Here's how the part is built. I have some questions about the finished solid (model axes, mm). Face numbers are marked on the shaded views. A direction names the side the tool comes from. Round coordinates to 2 decimals unless told otherwise and drop trailing zeros. Write each loop counter-clockwise with the first axis right and the second up, starting at its lowest first coordinate (ties: lowest second). Pieces come first, ordered by that corner, then holes. Notation, with made-up numbers: M -5,-27.75 L 23,-27.75 A15 cw 23,-2.75 Z; hole C -6,31 d1. An arc over 180 degrees is marked long. Use one line per item in the form item = value. Start each with the question number.
Q1. I want a section at A-A on x = -24.5. List the corners of the cut face in (y, z) for me.
Q2. I want a section at C-C on x = 5.5. List the corners of the cut face in (y, z) for me.
Q3. For the marked faces 1 and 2, which set-ups out of +Z, -Z, +X, -X, +Y, -Y let a thin tool reach every point of the face, with its end or its side?
Q4. I'm going to push flat-ended pins straight in: pin 1 Ø10 at (y, z) = (-18, 8) entering from -X; pin 2 Ø1 at (x, z) = (-18.5, 8.5) entering from +Y; pin 3 Ø10 at (x, y) = (-4.5, -1.5) entering from +Z. Where does each tip first touch, or does it pass through?
Q5. I want a section at D-D on z = 19.25. List the corners of the cut face in (x, y) for me, and give its area (3 significant figures).
Q6. I want a section at B-B on y = 1.5. List the corners of the cut face in (x, z) for me, and give its area (3 significant figures).
Q7. I need wall thicknesses on line 1 along Z through (x, y) = (-19, 15); line 2 along Y through (x, z) = (-9.5, 4). Which ranges of each line are inside material? Lowest first, please. Write a range as from..to.
```python
from build123d import *

# Parameters (mm, degrees)
SKETCH_1_W      = 40
SKETCH_1_H      = 70
EXTRUDE_1_DEPTH = 2
SKETCH_2_W      = 40
SKETCH_2_H      = 2
EXTRUDE_2_DEPTH = 20


with BuildPart() as part:
    # 草图1 → 凸台-拉伸1 (new body)
    with BuildSketch(Plane.XY):
        with Locations((-10.271445819, -4.719420773)):
            Rectangle(SKETCH_1_W, SKETCH_1_H)
        with BuildLine():
            Line((-25.271445819, -1.469420773), (-20.271445819, -1.469420773))
            Line((-20.271445819, -1.469420773), (-16.171194561, -1.469420773))
            ThreePointArc((-16.171194561, -1.469420773), (-11.103842793, 13.946987092), (3.728554181, 20.530579227))
            Line((3.728554181, 20.530579227), (3.728554181, 24.613768385))
            ThreePointArc((3.728554181, 24.613768385), (-12.578401723, 18.252971536), (-20.271445819, 2.530579227))
            Line((-20.271445819, 2.530579227), (-25.271445819, 2.530579227))
            ThreePointArc((-25.271445819, 2.530579227), (-27.271445819, 0.530579227), (-25.271445819, -1.469420773))
        make_face(mode=Mode.SUBTRACT)
    extrude(amount=EXTRUDE_1_DEPTH)

    # 草图2 → 凸台-拉伸2 (add)
    with BuildSketch(Plane.XY.offset(2)):
        with Locations((-10.271445819, -38.719420773)):
            Rectangle(SKETCH_2_W, SKETCH_2_H)
    extrude(amount=EXTRUDE_2_DEPTH)


solid = part.part
```
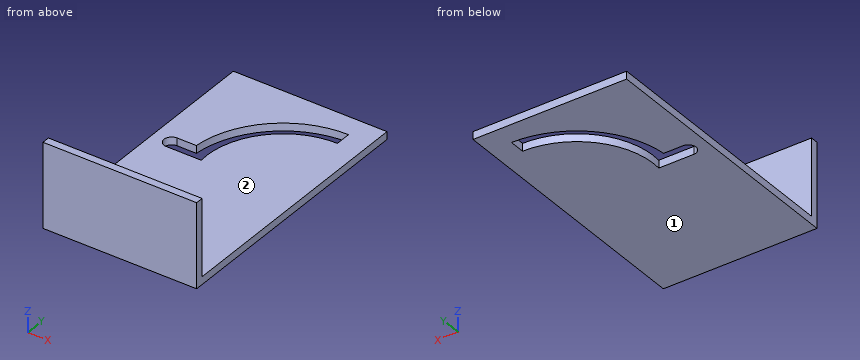
Reported:
q1.outline = M -39.72,0 L -1.47,0 L -1.47,2 L -37.72,2 L -37.72,22 L -39.72,22 Z; M 2.53,0 L 30.28,0 L 30.28,2 L 2.53,2 Z
q2.outline = M -39.72,0 L 30.28,0 L 30.28,2 L -37.72,2 L -37.72,22 L -39.72,22 Z
q3.face_1 = -Z, +X, -X, +Y, -Y
q3.face_2 = +Z, +X, -X, +Y
q4.pin_1 = through
q4.pin_2 = -37.72
q4.pin_3 = 2
q5.outline = M -30.27,-39.72 L 9.73,-39.72 L 9.73,-37.72 L -30.27,-37.72 Z
q5.area = 80.0 mm^2
q6.outline = M -30.27,0 L -27.02,0 L -27.02,2 L -30.27,2 Z; M -16.25,0 L 9.73,0 L 9.73,2 L -16.25,2 Z
q6.area = 58.5 mm^2
q7.line_1 = 0..2
q7.line_2 = -39.72..-37.72
